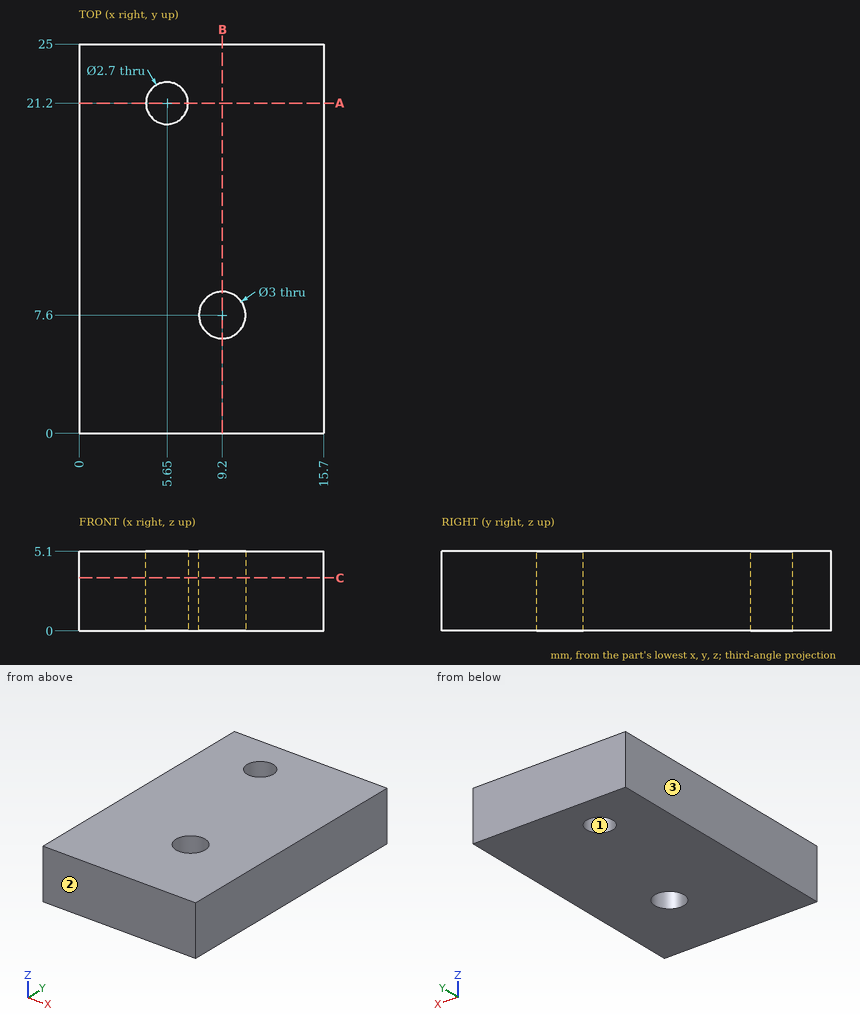
Design review of the part shown in the three views and the two pictorial views. Dimensions are in mm from the part's minimum x, y and z. Round coordinates to 2 decimals unless told otherwise and drop trailing zeros. Write each loop counter-clockwise with the first axis right and the second up, starting at its lowest first coordinate (ties: lowest second). Pieces come first, ordered by that corner, then holes.
Item 1: We need section C-C on z = 3.4. Write out the cut boundary in (x, y).
Item 2: The part is to be moulded in two halves that separate along X. For the marked faces 1, 2 and 3, say which applies: +X half, -X half, draft (parallel to the pull), parting line (faces both ways), or undercut.
Item 3: Clearance check with a flat-ended pin moving along its axis: pin 1 Ø2 at (x, z) = (7.5, 4) entering from -Y. State where the tip first meets the part, or that it passes through.
Item 4: We need section B-B on x = 9.2. Write out the cut boundary in (y, z), and give its area (3 significant figures).
Item 5: We need section A-A on y = 21.2. Write out the cut boundary in (x, z).
Item 6: For probe 1 along Y at (x, z) = (9.2, 2.05); probe 2 along Y at (x, z) = (5.65, 1.35); probe 3 along X at (y, z) = (20.25, 0.75), list the stretches that pass through material, from the lowest coordinate up.
Returned:
1. outline: (0, 0) - (15.7, 0) - (15.7, 25) - (0, 25) - close; hole circle Ø2.7 at (5.65, 21.2); hole circle Ø3 at (9.2, 7.6)
2. face 1: undercut
2. face 2: draft
2. face 3: -X half
3. pin 1: stops at y = 0
4. outline: (0, 0) - (6.1, 0) - (6.1, 5.1) - (0, 5.1) - close; (9.1, 0) - (25, 0) - (25, 5.1) - (9.1, 5.1) - close
4. area: 112 mm2
5. outline: (0, 0) - (4.3, 0) - (4.3, 5.1) - (0, 5.1) - close; (7, 0) - (15.7, 0) - (15.7, 5.1) - (7, 5.1) - close
6. probe 1: y = 0 to 6.1, 9.1 to 25
6. probe 2: y = 0 to 19.85, 22.55 to 25
6. probe 3: x = 0 to 4.69, 6.61 to 15.7
